The listing builds one solid part. Answer for the finished solid, in the listing's coordinates (mm). Round coordinates to 2 decimals unless told otherwise and drop trailing zeros. Loops run counter-clockwise (first coordinate to the right, second up) from the corner with the lowest first, then second, coordinate; pieces in that order, holes last. Notation, with made-up numbers: M 49.5,-8 L 76.5,-8 A21 ccw 76.5,-4 Z; hole C -5,10 d6. An arc over 180 degrees is marked long. Answer as a JSON object with one key per item and string values.
```python
from build123d import *

# Parameters (mm, degrees)
SKETCH1_R                = 38.1381
SKETCH1_R_2              = 36.5125
BOSS_EXTRUDE1_DEPTH      = 147.32
SHEAR_PIN_CUT_REACH      = 175.322
SHEAR_PIN_CUT_END_RADIUS = 36.5125
SKETCH2_R                = 0.9906
SHEAR_PIN_PATTERN_COUNT  = 3


with BuildPart() as part:
    # Sketch1 → Boss-Extrude1 (new body)
    with BuildSketch(Plane(origin=(0, 0, 0), x_dir=(1, 0, 0), z_dir=(0, 1, 0))):
        with Locations(Location((0, 0, 0), (0, 0, 270))):
            Circle(SKETCH1_R)
        with Locations(Location((0, 0, 0), (0, 0, 270))):
            Circle(SKETCH1_R_2, mode=Mode.SUBTRACT)
    extrude(amount=BOSS_EXTRUDE1_DEPTH)

    # Shear Pin Cut: up to this cylinder (the profile starts outside it)
    shear_pin_cut_end = Plane(origin=(0, 36.7284, 0), z_dir=(0, -1, 0)) * Cylinder(SHEAR_PIN_CUT_END_RADIUS, 424.669, mode=Mode.PRIVATE)
    # Sketch2 → Shear Pin Cut (cut, up to the surface)
    with BuildSketch(Plane(origin=(33.028563452, 0, 19.06905), x_dir=(0, -1, 0), z_dir=(0.866025403784438, 0, 0.500000000000001)), mode=Mode.PRIVATE) as shear_pin_cut_sk1:
        with Locations(Location((-36.7284, 0, 0), (0, 0, 90))):
            Circle(SKETCH2_R)
    shear_pin_cut_tool1 = extrude(shear_pin_cut_sk1.sketch, amount=-SHEAR_PIN_CUT_REACH, mode=Mode.PRIVATE) - shear_pin_cut_end
    shear_pin_cut = shear_pin_cut_tool1.solids().sort_by_distance((33.028563, 36.7284, 19.06905))[0]
    add(shear_pin_cut, mode=Mode.SUBTRACT)

    # Shear Pin Pattern: Shear Pin Cut ×3 about axis
    shear_pin_pattern_axis = Axis((0, 155.08605, 0), (0, -1, 0))
    for i in range(1, SHEAR_PIN_PATTERN_COUNT):
        add(shear_pin_cut.rotate(shear_pin_pattern_axis, i * 360 / SHEAR_PIN_PATTERN_COUNT), mode=Mode.SUBTRACT)


solid = part.part
```
Item 1: Straight lines are drawn through the part: line 1 (Z direction, x = 1, y = 56); line 2 (X direction, y = 37, z = 0); line 3 (Z direction, x = 33, y = 26). For each, find the intervals that lie inside material, in ascending order.
Values follow:
{"line 1": "-38.12 to -36.5, 36.5 to 38.12", "line 2": "-38.14 to -36.51, 36.51 to 38.14", "line 3": "-19.12 to -15.63, 15.63 to 19.12"}
Item 2: Flat-ended cylindrical pins translate along their axes: P1, Ø12, axis at y = 55, z = -10, coming from the +X side; P2, Ø1, axis at x = -2, y = 109, coming from the +Z side; P3, Ø6, axis at y = 46.5, z = -14.5, coming from the -X side. Find the tip coordinate at first contact, or state that the pin passes through.
Values follow:
{"P1": "x = 37.93", "P2": "z = 38.11", "P3": "x = -36.36"}
Item 3: The part is cut by section A-A (z = 0). Give the vertices of the cut face in (x, y), then the cut area to 3 significant figures.
Values follow:
{"outline": "M -38.14,0 L -36.51,0 L -36.51,147.32 L -38.14,147.32 Z; M 36.51,0 L 38.14,0 L 38.14,147.32 L 36.51,147.32 Z", "area": "479 mm^2"}
Item 4: The part is cut by section C-C (y = 128). Give the vertices of the cut face in (x, z) (1 decimal).
Values follow:
{"outline": "C 0,0 d76.3; hole C 0,0 d73"}
Item 5: The part is cut by section B-B (x = -13.5). Give the vertices of the cut face in (y, z).
Values follow:
{"outline": "M 0,-35.67 L 147.32,-35.67 L 147.32,-33.93 L 0,-33.93 Z; M 0,33.93 L 147.32,33.93 L 147.32,35.67 L 0,35.67 Z"}
